Could you check a few things on this model? Use its own coordinates, in mm. A direction names the side the tool comes from. Coordinates: 2 decimals unless noted, no trailing zeros. Order: outer loops, then holes, each group sorted by start corner. A loop starts at its lowest first (then second) coordinate and runs counter-clockwise, first axis right, second up. Notation, with made-up numbers: (22.25, 69) - (38.25, 69) arc R11 ccw to (38.25, 78) - close; hole circle Ø2 at (88, 82). An arc over 180 degrees is marked (long way). Answer as a JSON object with one key per item and string values. Group by question number.
(1) Will these pins go through, and if not, where does the flat tip stop? P1, Ø9.5, axis at x = 3, z = 22.5, coming from the +Y side; P2, Ø4, axis at x = 4.35, z = 5, coming from the +Y side; P3, Ø1.6, axis at y = 1, z = 20.5, coming from the +X side.
(2) Imagine slicing it at B-B, the plane x = 20. Write out the boundary of the cut face in (y, z).
(3) Please list where these lines run through material, in increasing order: probe 1 along Z at (x, y) = (49.5, 6.75); probe 2 along Y at (x, z) = (5, 31); probe 3 along Y at (x, z) = (12.5, 27.5).
(4) Which directions (+Z, -Z, +X, -X, +Y, -Y) give clear straight access to the entire face, cutting with the end or side of a thin tool? Please do faces 1 (the flat face through (4, 1.3, 37)), 2 (the flat face through (26.336, 5.273, 7.395)), 3 (the flat face through (52.88, 5.11, 32.39)).
(5) Imagine slicing it at C-C, the plane z = 14. Write out the boundary of the cut face in (x, y).
(6) Imagine slicing it at A-A, the plane z = 35. Write out the boundary of the cut face in (x, y).
(7) We'd pull the mould along X, two halves only. Please class faces 4 (the flat face through (8.702, 1, 20)), 5 (the flat face through (0, 1, 20)), 6 (the flat face through (4, 0, 20)), 7 (the cylindrical face through (2.79, 0.66, 4.65)): pulls with the +X half, pulls with the -X half, needs draft (parallel to the pull), parting line crosses it, or undercut.
from build123d import *

# Parameters (mm, degrees)
EXTRUDE_1_DEPTH                 = 40
FILLET_1_R                      = 10
CHAMFER_1_SIZE                  = 2
CHAMFER_1_SIZE_2                = 1.558687347
CUT_EXTRUDE_1_REACH             = 74.003
SKETCH_2_R                      = 1.6
SKETCH_3_R                      = 4
CUT_EXTRUDE_2_DEPTH             = 0.2
CUT_EXTRUDE_3_REACH             = 74.003
SKETCH_4_W                      = 50.702932162
SKETCH_4_H                      = 10
CUT_EXTRUDE_3_DIRECTION_2_REACH = 74.003


with BuildPart() as part:
    # 草图1 → 凸台-拉伸1 (new body)
    with BuildSketch(Plane.XY):
        Polygon((0, 0), (10, 0), (45, 8), (60, 2.5), (60, 3.565103021), (44.204382552, 9.356829418), (9.830753848, 1.5), (0, 1.5), align=None)
    extrude(amount=EXTRUDE_1_DEPTH)

    # 圆角1
    fillet_1_edges = [part.edges().sort_by_distance(p)[0] for p in [
        (9.830753848, 1.5, 20),
        (44.204382552, 9.356829418, 20),
        (45, 8, 20),
        (10, 0, 20),
    ]]
    fillet(fillet_1_edges, radius=FILLET_1_R)

    # 倒角1
    # the kernel refuses this chamfer: 2, 1.558687347 mm, written as the material it takes off along each edge
    with BuildSketch(Plane(origin=(60, 2.5, -5.143365976), x_dir=(-0.9479869259850683, 0.31830926496314954, 0), z_dir=(0, 0, 1))) as chamfer_1_piece_1:
        Polygon((CHAMFER_1_SIZE * 0.999621916911, -CHAMFER_1_SIZE * 0.0274958766106), (CHAMFER_1_SIZE_2 * 0.318309265001, -CHAMFER_1_SIZE_2 * 0.947986926099), (0, 0), align=None)
    extrude(amount=50.286731952, mode=Mode.SUBTRACT)

    # 草图2 → 切除-拉伸1 (cut, up to next)
    with BuildSketch(Plane(origin=(0, 1.5, 0), x_dir=(1, 0, 0), z_dir=(0, 1, 0)), mode=Mode.PRIVATE) as cut_extrude_1_sk1:
        with Locations(Location((4.351223085, -5, 0), (0, 0, 270))):
            Circle(SKETCH_2_R)
    cut_extrude_1_tool1 = extrude(cut_extrude_1_sk1.sketch, amount=-CUT_EXTRUDE_1_REACH, mode=Mode.PRIVATE) & part.part
    # 草图2 → 切除-拉伸1 (cut, up to next)
    with BuildSketch(Plane(origin=(0, 1.5, 0), x_dir=(1, 0, 0), z_dir=(0, 1, 0)), mode=Mode.PRIVATE) as cut_extrude_1_sk2:
        with Locations(Location((4.351223085, -35, 0), (0, 0, 270))):
            Circle(SKETCH_2_R)
    cut_extrude_1_tool2 = extrude(cut_extrude_1_sk2.sketch, amount=-CUT_EXTRUDE_1_REACH, mode=Mode.PRIVATE) & part.part
    add(cut_extrude_1_tool1.solids().sort_by_distance((4.351223, 1.5, 5))[0], mode=Mode.SUBTRACT)
    add(cut_extrude_1_tool2.solids().sort_by_distance((4.351223, 1.5, 35))[0], mode=Mode.SUBTRACT)

    # 草图3 → 切除-拉伸2 (cut)
    with BuildSketch(Plane(origin=(0, 1.5, 0), x_dir=(1, 0, 0), z_dir=(0, 1, 0))):
        with Locations(Location((4.351223085, -5, 0), (0, 0, 270))):
            Circle(SKETCH_3_R)
        with Locations(Location((4.351223085, -35, 0), (0, 0, 270))):
            Circle(SKETCH_3_R)
    extrude(amount=-CUT_EXTRUDE_2_DEPTH, mode=Mode.SUBTRACT)

    # 草图4 → 切除-拉伸3 (cut, up to next)
    with BuildSketch(Plane(origin=(0, 1.5, 0), x_dir=(1, 0, 0), z_dir=(0, 1, 0)), mode=Mode.PRIVATE) as cut_extrude_3_sk1:
        with Locations((34.053912252, -20)):
            Rectangle(SKETCH_4_W, SKETCH_4_H)
    cut_extrude_3_tool1 = extrude(cut_extrude_3_sk1.sketch, amount=-CUT_EXTRUDE_3_REACH, mode=Mode.PRIVATE) & part.part
    add(cut_extrude_3_tool1.solids().sort_by_distance((34.053912, 1.5, 20))[0], mode=Mode.SUBTRACT)

    # 草图4 → 切除-拉伸3 direction 2 (cut, up to next)
    with BuildSketch(Plane(origin=(0, 1.5, 0), x_dir=(1, 0, 0), z_dir=(0, 1, 0)), mode=Mode.PRIVATE) as cut_extrude_3_direction_2_sk1:
        with Locations((34.053912252, -20)):
            Rectangle(SKETCH_4_W, SKETCH_4_H)
    cut_extrude_3_direction_2_tool1 = extrude(cut_extrude_3_direction_2_sk1.sketch, amount=CUT_EXTRUDE_3_DIRECTION_2_REACH, mode=Mode.PRIVATE) & part.part
    add(cut_extrude_3_direction_2_tool1.solids().sort_by_distance((34.053912, 1.5, 20))[0], mode=Mode.SUBTRACT)


solid = part.part
Result set:
{
 "1": {"P1": "stops at y = 1.5", "P2": "stops at y = 1.3", "P3": "stops at x = 8.7"},
 "2": {"outline": "(2.29, 0) - (3.82, 0) - (3.82, 15) - (2.29, 15) - close; (2.29, 25) - (3.82, 25) - (3.82, 40) - (2.29, 40) - close"},
 "3": {"probe 1": "z = 0 to 15, 25 to 40", "probe 2": "y = 0 to 1.5", "probe 3": "y = 0.57 to 2.11"},
 "4": {"face 1": "+Y", "face 2": "+Z, -Z, -X, +Y", "face 3": "+Z, -Z, -Y"},
 "5": {"outline": "(0, 0) - (8.87, 0) arc R10 ccw to (11.1, 0.25) - (42.11, 7.34) arc R10 cw to (47.78, 6.98) - (58.12, 3.19) - (59.41, 3.78) - (46.99, 8.34) arc R10 ccw to (41.32, 8.7) - (10.93, 1.75) arc R10 cw to (8.7, 1.5) - (0, 1.5) - close"},
 "6": {"outline": "(0, 0) - (2.75, 0) - (2.75, 1.3) - (0.35, 1.3) - (0.35, 1.5) - (0, 1.5) - close; (5.95, 0) - (8.87, 0) arc R10 ccw to (11.1, 0.25) - (42.11, 7.34) arc R10 cw to (47.78, 6.98) - (58.12, 3.19) - (59.41, 3.78) - (46.99, 8.34) arc R10 ccw to (41.32, 8.7) - (10.93, 1.75) arc R10 cw to (8.7, 1.5) - (8.35, 1.5) - (8.35, 1.3) - (5.95, 1.3) - close"},
 "7": {"face 4": "pulls with the +X half", "face 5": "pulls with the -X half", "face 6": "needs draft", "face 7": "undercut"}
}
